```python
from build123d import *

# Parameters (mm, degrees)
BOSS_EXTRUDE1_DEPTH      = 40
BOSS_EXTRUDE1_DEPTH_BACK = 16
BOSS_EXTRUDE2_START      = -5
SKETCH1_3_R              = 52.187837327
BOSS_EXTRUDE2_DEPTH      = 11
CUT_EXTRUDE1_DEPTH       = 57
CUT_EXTRUDE3_DEPTH       = 40
CUT_EXTRUDE4_DEPTH       = 85.187837327
FILLET1_R                = 2
F_10_0MM_DOWEL_HOLE1_D   = 10
F_10_0MM_DOWEL_HOLE2_D   = 10
FILLET2_R                = 2
FILLET3_R                = 2


with BuildPart() as part:
    # Sketch1 → Boss-Extrude1 (new body, two sides)
    with BuildSketch(Plane.XY) as boss_extrude1_sk:
        with BuildLine():
            Line((-32, 0), (-32, 52.187837327))
            ThreePointArc((-32, 52.187837327), (0, 84.187837327), (32, 52.187837327))
            Line((32, 52.187837327), (32, 0))
            ThreePointArc((32, 0), (0, -32), (-32, 0))
        make_face()
    extrude(amount=BOSS_EXTRUDE1_DEPTH)
    extrude(boss_extrude1_sk.sketch, amount=-BOSS_EXTRUDE1_DEPTH_BACK)

    # Sketch1_3 → Boss-Extrude2 (add)
    with BuildSketch(Plane.XY.offset(BOSS_EXTRUDE2_START)):
        Circle(SKETCH1_3_R)
    extrude(amount=-BOSS_EXTRUDE2_DEPTH)

    # Sketch2 → Cut-Extrude1 (cut, through all)
    with BuildSketch(Plane.XY.offset(40)):
        with BuildLine():
            Line((-12.5, 0), (-12.5, 50))
            ThreePointArc((-12.5, 50), (0, 62.5), (12.5, 50))
            Line((12.5, 50), (12.5, 0))
            ThreePointArc((12.5, 0), (0, -12.5), (-12.5, 0))
        make_face()
    extrude(amount=-CUT_EXTRUDE1_DEPTH, mode=Mode.SUBTRACT)

    # Sketch6 → Cut-Extrude3 (cut)
    with BuildSketch(Plane.XY.offset(40)):
        with BuildLine():
            Line((-22, 0), (-22, 50))
            ThreePointArc((-22, 50), (0, 72), (22, 50))
            Line((22, 50), (22, 0))
            ThreePointArc((22, 0), (0, -22), (-22, 0))
        make_face()
    extrude(amount=-CUT_EXTRUDE3_DEPTH, mode=Mode.SUBTRACT)

    # Sketch7 → Cut-Extrude4 (cut, through all)
    with BuildSketch(Plane(origin=(32, 0, 0), x_dir=(0, 0, -1), z_dir=(1, 0, 0))):
        Polygon((0, 52.187837327), (0, 84.187837327), (-40, 84.187837327), (-40, 12), align=None)
    extrude(amount=-CUT_EXTRUDE4_DEPTH, mode=Mode.SUBTRACT)

    # Fillet1
    fillet1_edges = [part.edges().sort_by_distance(p)[0] for p in [
        (-27, 12, 40),
        (27, 12, 40),
    ]]
    fillet(fillet1_edges, radius=FILLET1_R)

    # 10.0mm Dowel Hole1 (through all)
    with Locations(Plane.XY):
        with Locations((-19.052558883, 61), (19.052558883, 61), (0, 72)):
            Hole(F_10_0MM_DOWEL_HOLE1_D / 2)

    # 10.0mm Dowel Hole2 (through all)
    with Locations(Plane(origin=(0, 0, -16), x_dir=(-1, 0, 0), z_dir=(0, 0, -1))):
        with Locations((0, -41), (41, 0), (-41, 0)):
            Hole(F_10_0MM_DOWEL_HOLE2_D / 2)

    # Fillet2
    fillet2_edges = [part.edges().sort_by_distance(p)[0] for p in [
        (-26.945471299, 52.187837327, 0),
        (26.945471299, 52.187837327, 0),
    ]]
    fillet(fillet2_edges, radius=FILLET2_R)

    # Fillet3
    fillet3_edges = [part.edges().sort_by_distance(p)[0] for p in [
        (-32, 41.225845835, -10.5),
        (32, 41.225845835, -10.5),
    ]]
    fillet(fillet3_edges, radius=FILLET3_R)


solid = part.part
```
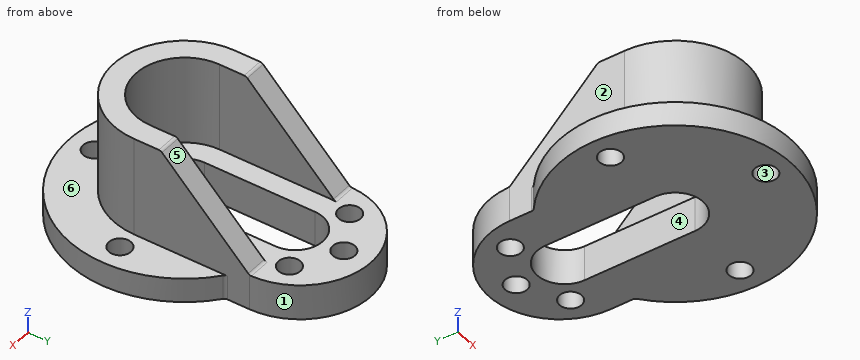
Part model, mm, in its own coordinate system. Face numbers are marked on the shaded views. A direction names the side the tool comes from. Round coordinates to 2 decimals unless told otherwise and drop trailing zeros. Loops run counter-clockwise (first coordinate to the right, second up) from the corner with the lowest first, then second, coordinate; pieces in that order, holes last.
1. 3-axis set-ups, long thin cutter, end or side, ignore diameter. For the marked faces 4, 5 and 6: which of +Z, -Z, +X, -X, +Y, -Y reach the whole face in a straight line?
Solutions:
face 4: +Z, -Z
face 5: +Z, +X, -X, +Y
face 6: +Z, -Y
2. Slice it at C-C (z = 9). Give the cut face in (x, y), and give its area (3 significant figures).
Solutions:
outline: (-32, 0) arc R32 ccw to (32, 0) - (32, 43.15) - (22, 43.15) - (22, 0) arc R22 cw to (-22, 0) - (-22, 43.15) - (-32, 43.15) - close
area: 1,710 mm2
3. Two-plate mould, pull along Y, no slides. Class the marked faces 1, 2 and 3: pulls with the +Y half, pulls with the -Y half, needs draft (parallel to the pull), parting line crosses it, or undercut.
Solutions:
face 1: pulls with the +Y half
face 2: needs draft
face 3: undercut
4. Flat gauge pins, fed straight in: pin 1 (8 mm diameter, centred on y = 36, z = -6.5, fed in from +X); pin 2 (2 mm diameter, centred on x = 28, z = 30.5, fed in from -Y); pin 3 (1.5 mm diameter, centred on x = 40, z = -7.5, fed in from -Y); pin 4 (6 mm diameter, centred on x = 0, y = 72, fed in from -Z). Where does each tip first touch, or does it go through?
Solutions:
pin 1: stops at x = 41.23
pin 2: stops at y = -17.18
pin 3: stops at y = -34.39
pin 4: passes through
5. Slice it at A-A (y = 61). Give the cut face in (x, z).
Solutions:
outline: (-30.76, -16) - (-24.05, -16) - (-24.05, 0) - (-30.76, 0) - close; (-14.05, -16) - (-5.94, -16) - (-5.94, 0) - (-14.05, 0) - close; (5.94, -16) - (14.05, -16) - (14.05, 0) - (5.94, 0) - close; (24.05, -16) - (30.76, -16) - (30.76, 0) - (24.05, 0) - close
6. Drill centre lines: line 1 along Y through (x, z) = (0, -3); line 2 along Y through (x, z) = (0, -14); line 3 along Z through (x, y) = (-25.5, -39). Where is each one in solid material? Low to high.
Solutions:
line 1: y = -32 to -12.5, 62.5 to 67, 77 to 84.19
line 2: y = -52.19 to -46, -36 to -12.5, 62.5 to 67, 77 to 84.19
line 3: z = -16 to -5
7. Slice it at B-B (x = -8). Give the cut face in (y, z), and give its area (3 significant figures).
Solutions:
outline: (-51.57, -16) - (-9.6, -16) - (-9.6, 0) - (-20.49, 0) - (-20.49, 40) - (-30.98, 40) - (-30.98, -5) - (-51.57, -5) - close; (59.6, -16) - (83.17, -16) - (83.17, 0) - (59.6, 0) - close
area: 1,370 mm2
8. Slice it at D-D (x = 41). Give the cut face in (y, z), and give its area (3 significant figures).
Solutions:
outline: (-32.29, -16) - (-5, -16) - (-5, -5) - (-32.29, -5) - close; (5, -16) - (32.29, -16) - (32.29, -5) - (5, -5) - close
area: 600 mm2
